Check sheet for the drawn part. Datum: minimum x, y, z corner. Units: mm. A direction names the side the tool comes from. Round coordinates to 2 decimals unless told otherwise and drop trailing zeros. Write each loop counter-clockwise with the first axis right and the second up, starting at its lowest first coordinate (ties: lowest second). Pieces come first, ordered by that corner, then holes. Notation, with made-up numbers: M 71,-24.75 L 114,-24.75 A17 ccw 114,-11.75 Z; hole C 52,87.25 d6. An arc over 180 degrees is marked long. Use a Markdown table: item, result.
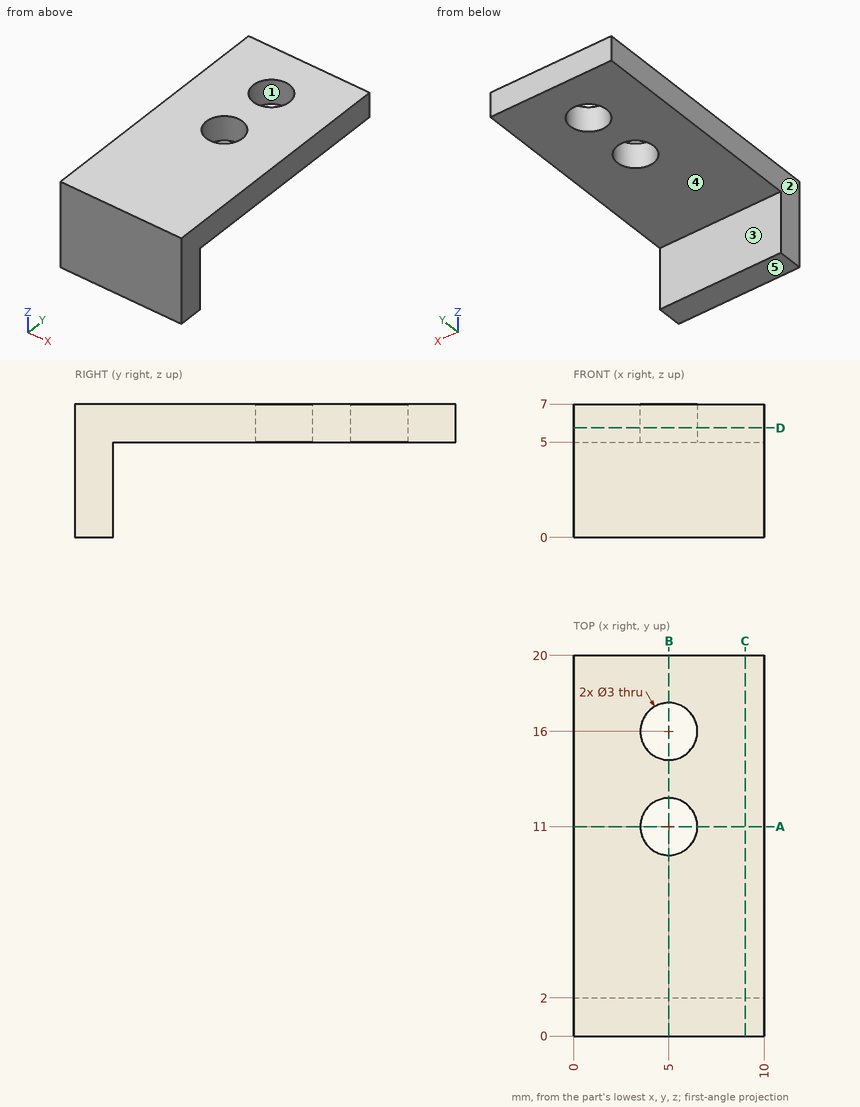
Item 1: Mould release check, pull along X, two halves, no side actions. Record for the marked faces 1, 2 and 3: +X half, -X half, draft (parallel to the pull), parting line (faces both ways), or undercut.
Outcome:
| item | result |
|---|---|
| face 1 | undercut |
| face 2 | -X half |
| face 3 | draft |
Item 2: Cross-section at C-C, the plane x = 9. Record the cut outline in (y, z), and give its area (3 significant figures).
Outcome:
| item | result |
|---|---|
| outline | M 0,0 L 2,0 L 2,5 L 20,5 L 20,7 L 0,7 Z |
| area | 50.0 mm2 |
Item 3: Access from +Z, -Z, +X, -X, +Y, -Y to the whole of each face (thin tool, end or side, straight path). Record for the marked faces 4 and 5.
Outcome:
| item | result |
|---|---|
| face 4 | -Z, +X, -X, +Y |
| face 5 | -Z, +X, -X, +Y, -Y |
Item 4: Cross-section at A-A, the plane y = 11. Record the cut outline in (x, z), and give its area (3 significant figures).
Outcome:
| item | result |
|---|---|
| outline | M 0,5 L 3.5,5 L 3.5,7 L 0,7 Z; M 6.5,5 L 10,5 L 10,7 L 6.5,7 Z |
| area | 14.0 mm2 |
Item 5: Cross-section at D-D, the plane z = 5.75. Record the cut outline in (x, y).
Outcome:
| item | result |
|---|---|
| outline | M 0,0 L 10,0 L 10,20 L 0,20 Z; hole C 5,11 d3; hole C 5,16 d3 |
Item 6: Cross-section at B-B, the plane x = 5. Record the cut outline in (y, z), and give its area (3 significant figures).
Outcome:
| item | result |
|---|---|
| outline | M 0,0 L 2,0 L 2,5 L 9.5,5 L 9.5,7 L 0,7 Z; M 12.5,5 L 14.5,5 L 14.5,7 L 12.5,7 Z; M 17.5,5 L 20,5 L 20,7 L 17.5,7 Z |
| area | 38.0 mm2 |
Item 7: Go/stop test with flat-tipped pins: pin 1 (5 mm diameter, centred on x = 5, y = 11, fed in from -Z); pin 2 (4 mm diameter, centred on x = 6.5, z = 2.5, fed in from +Y). Record where each tip stops, or that it passes through.
Outcome:
| item | result |
|---|---|
| pin 1 | stops at z = 5 |
| pin 2 | stops at y = 2 |
Item 8: Material ranges on line 1 along Y through (x, z) = (5, 6.3); line 2 along X through (y, z) = (11.25, 5.75); line 3 along Z through (x, y) = (8.5, 7.5), recorded low to high. Write a range as from..to.
Outcome:
| item | result |
|---|---|
| line 1 | y = 0..9.5, 12.5..14.5, 17.5..20 |
| line 2 | x = 0..3.52, 6.48..10 |
| line 3 | z = 5..7 |
